Read the model definition and answer for the solid it produces. Units are mm, in the model's axes. A direction names the side the tool comes from. Coordinates: 2 decimals unless noted, no trailing zeros. Write each loop counter-clockwise with the first axis right and the second up, starting at its lowest first coordinate (ties: lowest second). Pieces come first, ordered by that corner, then holes.
from build123d import *

# Parameters (mm, degrees)
SKETCH1_W           = 180
SKETCH1_H           = 75
BOSS_EXTRUDE1_DEPTH = 166
SKETCH2_W           = 50
SKETCH2_H           = 25
CUT_EXTRUDE1_DEPTH  = 15
FILLET1_R           = 2
SKETCH3_W           = 4
SKETCH3_H           = 15
BOSS_EXTRUDE2_DEPTH = 14
FILLET2_R           = 4


with BuildPart() as part:
    # Sketch1 → Boss-Extrude1 (new body)
    with BuildSketch(Plane(origin=(0, 0, 0), x_dir=(1, 0, 0), z_dir=(0, 1, 0))):
        Rectangle(SKETCH1_W, SKETCH1_H)
    extrude(amount=BOSS_EXTRUDE1_DEPTH)

    # Sketch2 → Cut-Extrude1 (cut)
    with BuildSketch(Plane.XZ):
        with Locations((-65, -25)):
            Rectangle(SKETCH2_W, SKETCH2_H)
        with Locations((65, -25)):
            Rectangle(SKETCH2_W, SKETCH2_H)
    extrude(amount=-CUT_EXTRUDE1_DEPTH, mode=Mode.SUBTRACT)

    # Fillet1
    fillet1_edges = [part.edges().sort_by_distance(p)[0] for p in [
        (0, 0, -37.5),
        (-90, 90.5, -37.5),
        (90, 90.5, -37.5),
        (90, 83, 37.5),
    ]]
    fillet(fillet1_edges, radius=FILLET1_R)

    # Sketch3 → Boss-Extrude2 (add)
    with BuildSketch(Plane.XZ.offset(-15)):
        with Locations((-72, -25)):
            Rectangle(SKETCH3_W, SKETCH3_H)
        with Locations((72, -25)):
            Rectangle(SKETCH3_W, SKETCH3_H)
    extrude(amount=BOSS_EXTRUDE2_DEPTH)

    # Fillet2
    fillet2_edges = [part.edges().sort_by_distance(p)[0] for p in [
        (-72, 1, -32.5),
        (-72, 1, -17.5),
        (72, 1, -17.5),
        (72, 1, -32.5),
    ]]
    fillet(fillet2_edges, radius=FILLET2_R)


solid = part.part
Item 1: Given pin 1 (4 mm diameter, centred on y = 10.5, z = -28, fed in from +X); pin 2 (2 mm diameter, centred on x = 71.5, y = 11, fed in from -Z); pin 3 (4.5 mm diameter, centred on x = 56, y = 8.5, fed in from -Z), each flat-ended and moving along its own axis, determine where each tip first touches the part or whether it passes through.
Item 2: The part is cut by section A-A (x = -77). Give the vertices of the cut face in (y, z).
Item 3: For faces 1 (the flat face through (-1, 0, 9)), 2 (the flat face through (-70, 8, -25)), 3 (the cylindrical face through (72.028, 2.203, -18.641)), 4 (the flat face through (74, 8, -25)), 5 (the cylindrical face through (-71.972, 2.203, -31.359)), determine the directions among +Z, -Z, +X, -X, +Y, -Y from which every point of the face is accessible in a straight line to the end or side of a thin tool.
Item 4: Determine the mould class of faces 6 (the flat face through (-72, 10, -32.5)), 7 (the cylindrical face through (-71.972, 2.203, -18.641)), 8 (the flat face through (40, 7, -25)), 9 (the flat face through (-72, 10, -17.5)) for opening direction Z: +Z half, -Z half, draft (parallel to the pull), parting line (faces both ways), or undercut.
Answer:
1. pin 1: stops at x = 74
1. pin 2: stops at z = -32.5
1. pin 3: stops at z = -12.5
2. outline: (0, -12.5) - (15, -12.5) - (15, -37.5) - (166, -37.5) - (166, 37.5) - (0, 37.5) - close
3. face 1: +Z, -Z, +X, -X, -Y
3. face 2: -Z, -Y
3. face 3: +X, -Y
3. face 4: -Z, +X, -Y
3. face 5: -Z, -X, -Y
4. face 6: -Z half
4. face 7: undercut
4. face 8: draft
4. face 9: undercut
